Geometry: final body of the model. Coordinates: model frame, mm. A direction names the side the tool comes from. Give positions to 0.01 mm unless a question says otherwise; leave off trailing zeros. Write each loop counter-clockwise with the first axis right and the second up, starting at its lowest first coordinate (ties: lowest second). Pieces come first, ordered by that corner, then holes. Notation, with made-up numbers: M -14.75,73.25 L -9.75,73.25 A35 cw -9.75,111.25 Z; hole C -9.5,42 d11. An arc over 180 degrees is marked long. Answer as a JSON object with one key per item and string values.
from build123d import *

# Parameters (mm, degrees)
SKETCH1_R               = 28
SKETCH1_R_2             = 16
BOSS_EXTRUDE1_DEPTH     = 56
SKETCH2_W               = 6
SKETCH2_H               = 44.450735801
CUT_EXTRUDE1_DEPTH      = 56
SKETCH3_W               = 48
SKETCH3_H               = 74
BOSS_EXTRUDE2_DEPTH     = 24
CUT_EXTRUDE4_DEPTH      = 134.489909528
CUT_EXTRUDE4_DEPTH_BACK = 40


with BuildPart() as part:
    # Sketch1 → Boss-Extrude1 (new body)
    with BuildSketch(Plane(origin=(0, 0, 0), x_dir=(1, 0, 0), z_dir=(0, 1, 0))):
        with Locations(Location((0, 0, 0), (0, 0, 270))):
            Circle(SKETCH1_R)
        with Locations(Location((0, 0, 0), (0, 0, 270))):
            Circle(SKETCH1_R_2, mode=Mode.SUBTRACT)
    extrude(amount=BOSS_EXTRUDE1_DEPTH)

    # Sketch2 → Cut-Extrude1 (cut)
    with BuildSketch(Plane(origin=(0, 56, 0), x_dir=(1, 0, 0), z_dir=(0, 1, 0))):
        with Locations((0.593322954, 8.717135315)):
            Rectangle(SKETCH2_W, SKETCH2_H)
    extrude(amount=-CUT_EXTRUDE1_DEPTH, mode=Mode.SUBTRACT)

    # Sketch3 → Boss-Extrude2 (add)
    with BuildSketch(Plane.XZ):
        with Locations((0, 53)):
            Rectangle(SKETCH3_W, SKETCH3_H)
    extrude(amount=-BOSS_EXTRUDE2_DEPTH)

    # Sketch4 → Cut-Extrude4 (cut, two sides: drawn at the far end of the back side and taken through both)
    with BuildSketch(Plane.XY.offset(90).offset(-CUT_EXTRUDE4_DEPTH_BACK)):
        with BuildLine():
            Line((-16, 142.81176407), (-16, 24))
            ThreePointArc((-16, 24), (0, 8), (16, 24))
            Line((16, 24), (16, 142.81176407))
            Line((16, 142.81176407), (16, 380.43529221))
            Line((16, 380.43529221), (-16, 380.43529221))
            Line((-16, 380.43529221), (-16, 142.81176407))
        make_face()
    extrude(amount=CUT_EXTRUDE4_DEPTH + CUT_EXTRUDE4_DEPTH_BACK, mode=Mode.SUBTRACT)


solid = part.part
1) Line query: line 1 (X direction, y = 15, z = 0); line 2 (Y direction, x = 5, z = 30.5); line 3 (Z direction, x = -7.5, y = 54). Output: solid intervals per line, ascending. Write a range as from..to.
Geometry check:
{"line 1": "x = -28..-16, 16..28", "line 2": "y = 0..24", "line 3": "z = -26.98..-14.13, 14.13..26.98"}
2) Cut plane A-A on z = 0. Return loops of the section in (x, y).
Geometry check:
{"outline": "M -28,0 L -16,0 L -16,56 L -28,56 Z; M 16,0 L 28,0 L 28,56 L 16,56 Z"}
3) Pull-direction query (X, two-part tool) for faces 1 (the cylindrical face through (0, 8, 70)), 2 (the flat face through (-24, 12, 52)), 3 (the flat face through (0, 6, 90)); classes: pulls with the +X half, pulls with the -X half, needs draft (parallel to the pull), parting line crosses it, or undercut.
Geometry check:
{"face 1": "undercut", "face 2": "pulls with the -X half", "face 3": "needs draft"}
4) Cut plane B-B on y = 14. Return loops of the section in (x, z).
Geometry check:
{"outline": "M -24,16 L -22.98,16 A28 ccw -2.41,-27.9 L -2.41,-15.82 A16 cw long 3.59,-15.59 L 3.59,-27.77 A28 ccw 22.98,16 L 24,16 L 24,90 L 12.49,90 L 12.49,50 L -12.49,50 L -12.49,90 L -24,90 Z"}
5) Contact query for flat-ended pins moving along their axis: P1, Ø3, axis at x = -14, y = 21, coming from the -Z side; P2, Ø6, axis at y = 21, z = -23.5, coming from the +X side; P3, Ø9.5, axis at y = 40.5, z = -23.5, coming from the -X side; P4, Ø3, axis at x = -11, z = 56.5, coming from the -Y side. Output: stop coordinate, or through.
Geometry check:
{"P1": "stops at z = -25.05", "P2": "stops at x = 19.07", "P3": "stops at x = -20.8", "P4": "stops at y = 0"}
6) Cut plane D-D on z = 69.5. Return loops of the section in (x, y), and give its area (3 significant figures).
Geometry check:
{"outline": "M -24,0 L 24,0 L 24,24 L 16,24 A16 cw -16,24 L -24,24 Z", "area": "750 mm2"}
7) Set-up query: faces 4 (the flat face through (0, 18, 50)), 5 (the flat face through (24, 12, 52)), 6 (the cylindrical face through (13.63, 27.61, -24.46)), 7 (the flat face through (-12, 56, 12)), 8 (the flat face through (3.593, 28, -22)). Return all of +Z, -Z, +X, -X, +Y, -Y with unobstructed straight access to the full face (end or side cutting, diameter ignored); none if empty.
Geometry check:
{"face 4": "+Z, +Y", "face 5": "+Z, +X, +Y, -Y", "face 6": "+Y", "face 7": "+Z, -Z, +X, -X, +Y", "face 8": "-Z, +Y, -Y"}
8) Cut plane C-C on x = 0. Return loops of the section in (y, z).
Geometry check:
{"outline": "M 0,16 L 56,16 L 56,28 L 24,28 L 24,50 L 8,50 L 8,90 L 0,90 Z"}
